Source: CAD feature listing. Evaluate the final solid. Frame: model axes, mm. A direction names the side the tool comes from. Give positions to 0.01 mm unless a question says otherwise; leave off trailing zeros. Order: outer loops, then holes, each group sorted by start corner. A loop starts at its lowest first (then second) coordinate and runs counter-clockwise, first axis right, second up.
from build123d import *

# Parameters (mm, degrees)
BOSS_EXTRUDE1_DEPTH      = 6.5
SKETCH5_R                = 3
SKETCH5_R_2              = 1.4
BOSS_EXTRUDE5_DEPTH      = 3.2
BOSS_EXTRUDE5_2_DEPTH    = 3.2
BOSS_EXTRUDE5_3_DEPTH    = 3.2
BOSS_EXTRUDE5_4_DEPTH    = 3.2
BOSS_EXTRUDE6_START      = -1.5
BOSS_EXTRUDE6_DEPTH      = 1.5
CUT_EXTRUDE9_START       = -1.5
SKETCH17_R               = 1.4
CUT_EXTRUDE9_DEPTH       = 1.5
CUT_EXTRUDE10_DEPTH      = 10
CUT_EXTRUDE10_DEPTH_BACK = 4
SKETCH18_W               = 118.483225972
SKETCH18_H               = 113.092379331
SKETCH19_W               = 5
SKETCH19_H               = 5
BOSS_EXTRUDE9_DEPTH      = 7
SKETCH20_R               = 1.4
BOSS_EXTRUDE10_DEPTH     = 1.3


with BuildPart() as part:
    # Sketch3 → Boss-Extrude1 (new body)
    with BuildSketch(Plane.XY.offset(55.290865561)):
        with BuildLine():
            Line((-23.272824317, 59.357808031), (-23.272824317, 9.357808031))
            ThreePointArc((-23.272824317, 9.357808031), (-21.808358223, 5.822274126), (-18.272824317, 4.357808031))
            Line((-18.272824317, 4.357808031), (40.727175683, 4.357808031))
            ThreePointArc((40.727175683, 4.357808031), (44.262709589, 5.822274126), (45.727175683, 9.357808031))
            Line((45.727175683, 9.357808031), (45.727175683, 59.357808031))
            ThreePointArc((45.727175683, 59.357808031), (44.262709589, 62.893341937), (40.727175683, 64.357808031))
            Line((40.727175683, 64.357808031), (-18.272824317, 64.357808031))
            ThreePointArc((-18.272824317, 64.357808031), (-21.808358223, 62.893341937), (-23.272824317, 59.357808031))
        make_face()
        with BuildLine():
            Line((40.727175683, 62.857808031), (-18.272824317, 62.857808031))
            ThreePointArc((-18.272824317, 62.857808031), (-20.747698051, 61.832681766), (-21.772824317, 59.357808031))
            Line((-21.772824317, 59.357808031), (-21.772824317, 9.357808031))
            ThreePointArc((-21.772824317, 9.357808031), (-20.747698051, 6.882934297), (-18.272824317, 5.857808031))
            Line((-18.272824317, 5.857808031), (40.727175683, 5.857808031))
            ThreePointArc((40.727175683, 5.857808031), (43.202049418, 6.882934297), (44.227175683, 9.357808031))
            Line((44.227175683, 9.357808031), (44.227175683, 59.357808031))
            ThreePointArc((44.227175683, 59.357808031), (43.202049418, 61.832681766), (40.727175683, 62.857808031))
        make_face(mode=Mode.SUBTRACT)
    extrude(amount=BOSS_EXTRUDE1_DEPTH)



with BuildPart() as body_2:
    # Sketch5 → Boss-Extrude5 (new body)
    with BuildSketch(Plane.XY.offset(55.290865561)):
        with Locations((-17.772824317, 58.857808031)):
            Circle(SKETCH5_R)
        with Locations(Location((-17.772824317, 58.857808031, 0), (0, 0, 180))):
            Circle(SKETCH5_R_2, mode=Mode.SUBTRACT)
    extrude(amount=BOSS_EXTRUDE5_DEPTH)


with BuildPart() as body_3:
    # Sketch5 → Boss-Extrude5 2 (new body)
    with BuildSketch(Plane.XY.offset(55.290865561)):
        with Locations(Location((40.227175683, 58.857808031, 0), (0, 0, 180))):
            Circle(SKETCH5_R)
        with Locations((40.227175683, 58.857808031)):
            Circle(SKETCH5_R_2, mode=Mode.SUBTRACT)
    extrude(amount=BOSS_EXTRUDE5_2_DEPTH)


with BuildPart() as body_4:
    # Sketch5 → Boss-Extrude5 3 (new body)
    with BuildSketch(Plane.XY.offset(55.290865561)):
        with Locations(Location((-17.772824317, 9.857808031, 0), (0, 0, 180))):
            Circle(SKETCH5_R)
        with Locations((-17.772824317, 9.857808031)):
            Circle(SKETCH5_R_2, mode=Mode.SUBTRACT)
    extrude(amount=BOSS_EXTRUDE5_3_DEPTH)


with BuildPart() as body_5:
    # Sketch5 → Boss-Extrude5 4 (new body)
    with BuildSketch(Plane.XY.offset(55.290865561)):
        with Locations((40.227175683, 9.857808031)):
            Circle(SKETCH5_R)
        with Locations(Location((40.227175683, 9.857808031, 0), (0, 0, 180))):
            Circle(SKETCH5_R_2, mode=Mode.SUBTRACT)
    extrude(amount=BOSS_EXTRUDE5_4_DEPTH)


with BuildPart() as part_1:
    add(part.part)

    add(body_2.part)  # Boss-Extrude6 merges body 2

    add(body_3.part)  # Boss-Extrude6 merges body 3

    add(body_4.part)  # Boss-Extrude6 merges body 4

    add(body_5.part)  # Boss-Extrude6 merges body 5
    # Sketch13 → Boss-Extrude6 (add)
    with BuildSketch(Plane.XY.offset(55.290865561).offset(BOSS_EXTRUDE6_START)):
        with BuildLine():
            Line((-23.272824317, 26.657808031), (-23.272824317, 42.657808031))
            Line((-23.272824317, 42.657808031), (-23.272824317, 59.357808031))
            ThreePointArc((-23.272824317, 59.357808031), (-21.808358223, 62.893341937), (-18.272824317, 64.357808031))
            Line((-18.272824317, 64.357808031), (40.727175683, 64.357808031))
            ThreePointArc((40.727175683, 64.357808031), (44.262709589, 62.893341937), (45.727175683, 59.357808031))
            Line((45.727175683, 59.357808031), (45.727175683, 9.357808031))
            ThreePointArc((45.727175683, 9.357808031), (44.262709589, 5.822274126), (40.727175683, 4.357808031))
            Line((40.727175683, 4.357808031), (-18.272824317, 4.357808031))
            ThreePointArc((-18.272824317, 4.357808031), (-21.808358223, 5.822274126), (-23.272824317, 9.357808031))
            Line((-23.272824317, 9.357808031), (-23.272824317, 26.657808031))
        make_face()
    extrude(amount=BOSS_EXTRUDE6_DEPTH)

    # Sketch17 → Cut-Extrude9 (cut)
    with BuildSketch(Plane.XY.offset(55.290865561).offset(CUT_EXTRUDE9_START)):
        with Locations(Location((40.227175683, 9.857808031, 0), (0, 0, 180))):
            Circle(SKETCH17_R)
        with Locations(Location((-17.772824317, 9.857808031, 0), (0, 0, 180))):
            Circle(SKETCH17_R)
        with Locations(Location((-17.772824317, 58.857808031, 0), (0, 0, 180))):
            Circle(SKETCH17_R)
        with Locations(Location((40.227175683, 58.857808031, 0), (0, 0, 180))):
            Circle(SKETCH17_R)
    extrude(amount=CUT_EXTRUDE9_DEPTH, mode=Mode.SUBTRACT)

    # Sketch18 → Cut-Extrude10 (cut, two sides: drawn at the far end of the back side and taken through both)
    with BuildSketch(Plane.XY.offset(58.490865561).offset(-CUT_EXTRUDE10_DEPTH_BACK)):
        with Locations((8.738192824, 45.025275568)):
            Rectangle(SKETCH18_W, SKETCH18_H)
    extrude(amount=CUT_EXTRUDE10_DEPTH + CUT_EXTRUDE10_DEPTH_BACK, mode=Mode.SUBTRACT)

    # Sketch19 → Boss-Extrude9 (add)
    with BuildSketch(Plane(origin=(0, 0, 53.790865561), x_dir=(-1, 0, 0), z_dir=(0, 0, -1))):
        with Locations((-33.227175683, 51.857808031)):
            Rectangle(SKETCH19_W, SKETCH19_H)
        with Locations((10.772824317, 16.857808031)):
            Rectangle(SKETCH19_W, SKETCH19_H)
        with Locations((10.772824317, 51.857808031)):
            Rectangle(SKETCH19_W, SKETCH19_H)
        with Locations((-33.227175683, 16.857808031)):
            Rectangle(SKETCH19_W, SKETCH19_H)
    extrude(amount=BOSS_EXTRUDE9_DEPTH)

    # Sketch20 → Boss-Extrude10 (add)
    with BuildSketch(Plane.XY.offset(54.490865561)):
        with BuildLine():
            Line((40.727175683, 64.357808031), (-18.272824317, 64.357808031))
            ThreePointArc((-18.272824317, 64.357808031), (-21.808358223, 62.893341937), (-23.272824317, 59.357808031))
            Line((-23.272824317, 59.357808031), (-23.272824317, 9.357808031))
            ThreePointArc((-23.272824317, 9.357808031), (-21.808358223, 5.822274126), (-18.272824317, 4.357808031))
            Line((-18.272824317, 4.357808031), (40.727175683, 4.357808031))
            ThreePointArc((40.727175683, 4.357808031), (44.262709589, 5.822274126), (45.727175683, 9.357808031))
            Line((45.727175683, 9.357808031), (45.727175683, 59.357808031))
            ThreePointArc((45.727175683, 59.357808031), (44.262709589, 62.893341937), (40.727175683, 64.357808031))
        make_face()
        with Locations(Location((-17.772824317, 9.857808031, 0), (0, 0, 180))):
            Circle(SKETCH20_R, mode=Mode.SUBTRACT)
        with Locations((-17.772824317, 58.857808031)):
            Circle(SKETCH20_R, mode=Mode.SUBTRACT)
        with Locations(Location((40.227175683, 58.857808031, 0), (0, 0, 180))):
            Circle(SKETCH20_R, mode=Mode.SUBTRACT)
        with Locations((40.227175683, 9.857808031)):
            Circle(SKETCH20_R, mode=Mode.SUBTRACT)
    extrude(amount=BOSS_EXTRUDE10_DEPTH)


solid = part_1.part
(1) Access query for faces 4 (the flat face through (-13.273, 17, 50)), 5 (the flat face through (-8.273, 52, 50)), 6 (the flat face through (-11, 14.358, 50)). Directions: +Z, -Z, +X, -X, +Y, -Y. A direction counts if a zero-diameter tool reaches every point of the face in a straight line with its end or side. Return the directions, or none.
(2) Pin query (flat end, axial travel): pin 1 Ø4.5 at (x, y) = (40.23, 9.86) entering from -Z; pin 2 Ø2.5 at (x, z) = (-10.5, 49) entering from +Y; pin 3 Ø4.5 at (x, y) = (40.23, 58.86) entering from +Z; pin 4 Ø4 at (y, z) = (17, 49) entering from +X. Return the tip coordinate at first contact, or that it passes through.
(3) Line query: line 1 along X through (y, z) = (54, 48.5); line 2 along Y through (x, z) = (-10.5, 47.75); line 3 along Y through (x, z) = (41, 54.75). Output: solid intervals per line, ascending.
(4) Section C-C, the plane x = 12. Return loops of the section in (y, z).
(5) Section A-A, the plane z = 53. Return loops of the section in (x, y).
(6) Section B-B, the plane y = 51.5. Return loops of the section in (x, z).
(7) Draft query along X for faces 1 (the cylindrical face through (44.301, 62.854, 54.777)), 2 (the flat face through (30.727, 17, 50)), 3 (the flat face through (33, 19.358, 50)). Return one class per face: +X half, -X half, draft (parallel to the pull), parting line (faces both ways), or undercut.
Checks:
1. face 4: -Z, -X, +Y, -Y
1. face 5: -Z, +Y, -Y
1. face 6: -Z, +X, -X, -Y
2. pin 1: stops at z = 53.79
2. pin 2: stops at y = 54.36
2. pin 3: stops at z = 55.79
2. pin 4: stops at x = 35.73
3. line 1: x = -13.27 to -8.27, 30.73 to 35.73
3. line 2: y = 14.36 to 19.36, 49.36 to 54.36
3. line 3: y = 4.37 to 8.69, 11.03 to 57.69, 60.03 to 64.35
4. outline: (4.36, 53.79) - (64.36, 53.79) - (64.36, 55.79) - (4.36, 55.79) - close
5. outline: (-13.27, 14.36) - (-8.27, 14.36) - (-8.27, 19.36) - (-13.27, 19.36) - close; (-13.27, 49.36) - (-8.27, 49.36) - (-8.27, 54.36) - (-13.27, 54.36) - close; (30.73, 14.36) - (35.73, 14.36) - (35.73, 19.36) - (30.73, 19.36) - close; (30.73, 49.36) - (35.73, 49.36) - (35.73, 54.36) - (30.73, 54.36) - close
6. outline: (-23.27, 53.79) - (-13.27, 53.79) - (-13.27, 46.79) - (-8.27, 46.79) - (-8.27, 53.79) - (30.73, 53.79) - (30.73, 46.79) - (35.73, 46.79) - (35.73, 53.79) - (45.73, 53.79) - (45.73, 55.79) - (-23.27, 55.79) - close
7. face 1: +X half
7. face 2: undercut
7. face 3: draft
